from build123d import *

# Parameters (mm, degrees)
SKETCH3_R                     = 11
BOSS_EXTRUDE1_DEPTH           = 10
SKETCH4_W                     = 73.6
SKETCH4_H                     = 48
SKETCH4_R                     = 9
BOSS_EXTRUDE2_DEPTH           = 2
CSK_FOR_M5_SFHCS1_D           = 5.3
CSK_FOR_M5_SFHCS1_CSINK_D     = 11.2
CSK_FOR_M5_SFHCS1_CSINK_ANGLE = 90
CHAMFER1_SIZE                 = 8
FILLET1_R                     = 4
FILLET2_R                     = 1.5
CSK_FOR_M3_SFHCS1_D           = 3.2
CSK_FOR_M3_SFHCS1_CSINK_D     = 6.72
CSK_FOR_M3_SFHCS1_CSINK_ANGLE = 90


with BuildPart() as part:
    # Sketch3 → Boss-Extrude1 (new body)
    with BuildSketch(Plane(origin=(0, 0, 0), x_dir=(1, 0, 0), z_dir=(0, 1, 0))):
        Polygon((-17, -17), (17, -17), (36.8, -17), (36.8, 11), (36.8, 31), (-36.8, 31), (-36.8, 11), (-36.8, -17), align=None)
        with Locations(Location((0, 0, 0), (0, 0, 270))):
            Circle(SKETCH3_R, mode=Mode.SUBTRACT)
    extrude(amount=BOSS_EXTRUDE1_DEPTH)

    # Sketch4 → Boss-Extrude2 (add)
    with BuildSketch(Plane(origin=(0, 10, 0), x_dir=(1, 0, 0), z_dir=(0, 1, 0))):
        with Locations((0, 7)):
            Rectangle(SKETCH4_W, SKETCH4_H)
        with Locations(Location((0, 0, 0), (0, 0, 270))):
            Circle(SKETCH4_R, mode=Mode.SUBTRACT)
    extrude(amount=BOSS_EXTRUDE2_DEPTH)

    # CSK for M5 SFHCS1 (through all)
    with Locations(Plane(origin=(0, 12, 0), x_dir=(1, 0, 0), z_dir=(0, 1, 0))):
        with Locations((26.8, 21), (-26.8, 21)):
            CounterSinkHole(CSK_FOR_M5_SFHCS1_D / 2, CSK_FOR_M5_SFHCS1_CSINK_D / 2, counter_sink_angle=CSK_FOR_M5_SFHCS1_CSINK_ANGLE)

    # Chamfer1
    chamfer1_edges = [part.edges().sort_by_distance(p)[0] for p in [
        (-36.8, 6, 17),
        (36.8, 6, 17),
    ]]
    chamfer(chamfer1_edges, length=CHAMFER1_SIZE)

    # Fillet1
    fillet1_edges = [part.edges().sort_by_distance(p)[0] for p in [
        (-36.8, 6, -31),
        (36.8, 6, -31),
        (28.8, 6, 17),
        (-28.8, 6, 17),
        (-36.8, 6, 9),
        (36.8, 6, 9),
    ]]
    fillet(fillet1_edges, radius=FILLET1_R)

    # Fillet2
    fillet2_edges = [part.edges().sort_by_distance(p)[0] for p in [
        (0, 12, -9),
        (-36.8, 0, -9.828427125),
        (-36.8, 12, -9.828427125),
        (0, 0, 17),
        (-32.8, 0, 13),
        (0, 0, -31),
        (36.8, 0, -9.828427125),
        (32.8, 0, 13),
        (-28.67387948, 0, 16.69551813),
        (-36.49551813, 0, 8.87387948),
        (28.67387948, 0, 16.69551813),
        (36.49551813, 0, 8.87387948),
        (35.628427125, 0, -29.828427125),
        (-35.628427125, 0, -29.828427125),
        (0, 12, -31),
        (-32.8, 12, 13),
        (0, 12, 17),
        (32.8, 12, 13),
        (36.8, 12, -9.828427125),
        (-28.67387948, 12, 16.69551813),
        (-36.49551813, 12, 8.87387948),
        (28.67387948, 12, 16.69551813),
        (36.49551813, 12, 8.87387948),
        (35.628427125, 12, -29.828427125),
        (-35.628427125, 12, -29.828427125),
    ]]
    fillet(fillet2_edges, radius=FILLET2_R)

    # CSK for M3 SFHCS1 (through all)
    with Locations(Plane(origin=(0, 12, 0), x_dir=(1, 0, 0), z_dir=(0, 1, 0))):
        with Locations((24.8, 5), (-24.8, 5)):
            CounterSinkHole(CSK_FOR_M3_SFHCS1_D / 2, CSK_FOR_M3_SFHCS1_CSINK_D / 2, counter_sink_angle=CSK_FOR_M3_SFHCS1_CSINK_ANGLE)


solid = part.part
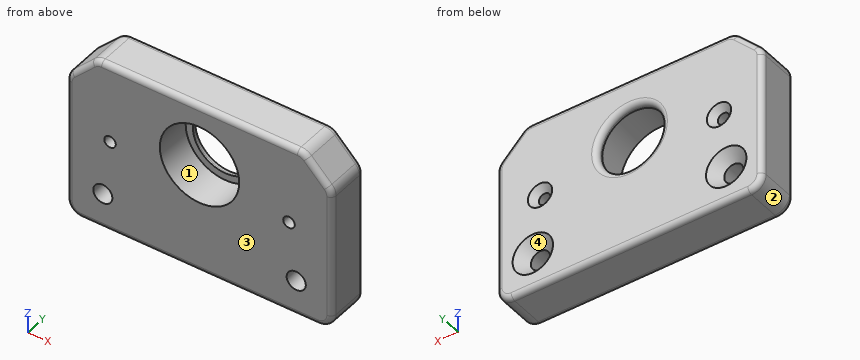
Read the model definition and answer for the solid it produces. Units are mm, in the model's axes. Face numbers are marked on the shaded views. Round coordinates to 2 decimals unless told otherwise and drop trailing zeros. Write each loop counter-clockwise with the first axis right and the second up, starting at its lowest first coordinate (ties: lowest second). Pieces come first, ordered by that corner, then holes.
Q1. The mould has two halves that part along Z. Classify the marked faces 1, 2, 3 and 4: released by +Z, released by -Z, zero draft, split by the parting line, or undercut.
Values:
face 1: undercut
face 2: released by -Z
face 3: zero draft
face 4: undercut
Q2. Find section B-B on z = -20. State how many separate pieces and enclosed holes the cut face has, and give its area (3 significant figures).
Values:
separate pieces: 3
enclosed holes: 0
area: 745 mm2
Q3. Find section A-A on y = 7.75. Determine the outline of the cut face in (x, z), and give its area (3 significant figures).
Values:
outline: (-36.8, -27) arc R4 ccw to (-32.8, -31) - (32.8, -31) arc R4 ccw to (36.8, -27) - (36.8, 7.34) arc R4 ccw to (35.63, 10.17) - (29.97, 15.83) arc R4 ccw to (27.14, 17) - (-27.14, 17) arc R4 ccw to (-29.97, 15.83) - (-35.63, 10.17) arc R4 ccw to (-36.8, 7.34) - close; hole circle Ø5.3 at (-26.8, -21); hole circle Ø3.2 at (-24.8, -5); hole circle Ø22 at (0, 0); hole circle Ø3.2 at (24.8, -5); hole circle Ø5.3 at (26.8, -21)
area: 3,020 mm2
Q4. Flat-ended cylindrical pins translate along their axes: P1, Ø3, axis at x = 24.8, z = -5, coming from the +Y side; P2, Ø20.5, axis at x = 0, z = 0, coming from the +Y side. Find the tip coordinate at first contact, or state that the pin passes through.
Values:
P1: passes through
P2: stops at y = 11.98
Q5. Straight lines are drawn through the part: line 1 (X direction, y = 6.5, z = -21); line 2 (Z direction, x = 24.8, y = 4); line 3 (X direction, y = 5.75, z = 0). For each, find the intervals that lie inside material, in ascending order.
Values:
line 1: x = -36.8 to -29.45, -24.15 to 24.15, 29.45 to 36.8
line 2: z = -31 to -22.74, -19.26 to -6.6, -3.4 to 17
line 3: x = -36.8 to -11, 11 to 36.8
